The drawing under review shows one solid part. Ordinate dimensions are in mm from its lowest x, y, z. Round coordinates to 2 decimals unless told otherwise and drop trailing zeros. Order: outer loops, then holes, each group sorted by start corner. A loop starts at its lowest first (then second) coordinate and runs counter-clockwise, first axis right, second up. Notation, with made-up numbers: (80, 67) -> (113, 67) arc R19 cw to (113, 84) -> close; hole circle Ø9 at (-19.75, 27.25). An arc over 180 degrees is marked (long way). Return JSON: item names as keys, results as strings. Group by question number.
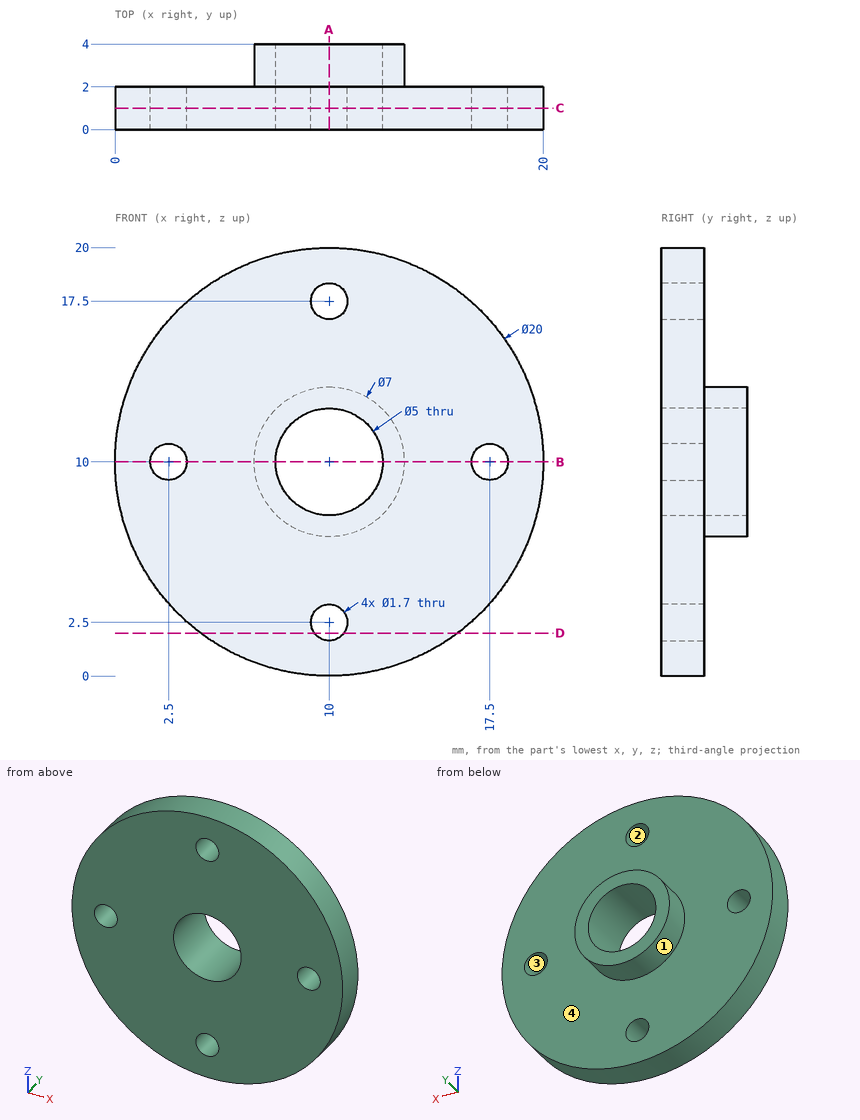
Item 1: Wall thickness on line 1 along Z through (x, y) = (9.25, 1.95); line 2 along X through (y, z) = (2.8, 10); line 3 along X through (y, z) = (1.15, 10): over which ranges is each line inside the solid? List them lowest first.
Item 2: Consider section D-D on z = 2. State the section outline as (x, y) points.
Item 3: Consider section B-B on z = 10. State the section outline as (x, y) points, plus the area to 3 significant figures.
Item 4: The part is to be moulded in two halves that separate along Z. For the marked faces 1, 2, 3 and 4, say which applies: +Z half, -Z half, draft (parallel to the pull), parting line (faces both ways), or undercut.
Item 5: Consider section C-C on y = 1. State the section outline as (x, z) points, plus the area to 3 significant figures.
Item 6: Consider section A-A on x = 10. State the section outline as (y, z) points, plus the area to 3 significant figures.
Item 7: Insertion check: pin 1 Ø4 at (x, z) = (16, 11) entering from +Y; pin 2 Ø6 at (x, z) = (9.5, 6) entering from +Y. Each pin has a flat end and moves straight along its axis. Give the tip position at first contact, or say it passes through.
Values:
{
 "1": {"line 1": "0.03 to 2.1, 2.9 to 7.62, 12.38 to 17.1, 17.9 to 19.97", "line 2": "6.5 to 7.5, 12.5 to 13.5", "line 3": "0 to 1.65, 3.35 to 7.5, 12.5 to 16.65, 18.35 to 20"},
 "2": {"outline": "(4, 0) -> (9.31, 0) -> (9.31, 2) -> (4, 2) -> close; (10.69, 0) -> (16, 0) -> (16, 2) -> (10.69, 2) -> close"},
 "3": {"outline": "(0, 0) -> (1.65, 0) -> (1.65, 2) -> (0, 2) -> close; (3.35, 0) -> (7.5, 0) -> (7.5, 4) -> (6.5, 4) -> (6.5, 2) -> (3.35, 2) -> close; (12.5, 0) -> (16.65, 0) -> (16.65, 2) -> (13.5, 2) -> (13.5, 4) -> (12.5, 4) -> close; (18.35, 0) -> (20, 0) -> (20, 2) -> (18.35, 2) -> close", "area": "27.2 mm^2"},
 "4": {"face 1": "parting line", "face 2": "undercut", "face 3": "undercut", "face 4": "draft"},
 "5": {"outline": "circle Ø20 at (10, 10); hole circle Ø1.7 at (2.5, 10); hole circle Ø5 at (10, 10); hole circle Ø1.7 at (10, 2.5); hole circle Ø1.7 at (10, 17.5); hole circle Ø1.7 at (17.5, 10)", "area": "285 mm^2"},
 "6": {"outline": "(0, 0) -> (2, 0) -> (2, 1.65) -> (0, 1.65) -> close; (0, 3.35) -> (2, 3.35) -> (2, 6.5) -> (4, 6.5) -> (4, 7.5) -> (0, 7.5) -> close; (0, 12.5) -> (4, 12.5) -> (4, 13.5) -> (2, 13.5) -> (2, 16.65) -> (0, 16.65) -> close; (0, 18.35) -> (2, 18.35) -> (2, 20) -> (0, 20) -> close", "area": "27.2 mm^2"},
 "7": {"pin 1": "y = 2", "pin 2": "y = 4"}
}
